Source: CAD feature listing. Evaluate the final solid. Frame: model axes, mm. A direction names the side the tool comes from. Give positions to 0.01 mm unless a question says otherwise; leave off trailing zeros. Write each loop counter-clockwise with the first axis right and the second up, starting at its lowest first coordinate (ties: lowest second). Pieces come first, ordered by that corner, then holes. Notation, with made-up numbers: (46.25, 7) -> (70.25, 7) arc R20 ccw to (70.25, 12) -> close; hole circle Ø3 at (89.5, 79.25). An arc over 180 degrees is marked (long way). Answer as a JSON object with one key per item and string values. Group by question number.
Item 1: Pull-direction query (X, two-part tool) for faces 1 (the face through (0, 15, 33)), 2 (the face through (-25, 0, 50)), 3 (the face through (-14.985, -0.66, 14.79)); classes: pulls with the +X half, pulls with the -X half, needs draft (parallel to the pull), parting line crosses it, or undercut.
Item 2: Section query D-D on z = 26. Return the cut outline in (x, y), plus the area to 3 significant figures.
Item 3: Access query for faces 4 (the face through (0, 0, 35)), 5 (the face through (-30, 0, 47)), 6 (the face through (21, 0, 30)). Directions: +Z, -Z, +X, -X, +Y, -Y. A direction counts if a zero-diameter tool reaches every point of the face in a straight line with its end or side. Return the directions, or none.
Item 4: First-contact query: pin 1 Ø5 at (x, y) = (-18, -10.5) entering from -Z; pin 2 Ø2 at (x, y) = (-23.5, 10.5) entering from +Z. Flat tips, straight axial feed; report the tip coordinate or a pass-through.
Item 5: Section query C-C on x = -14. Return the cut outline in (y, z), plus the area to 3 significant figures.
Item 6: Section query A-A on z = 40. Return the cut outline in (x, y).
Item 7: Section query B-B on y = 0. Return the cut outline in (x, z).
Item 8: Ray query, probe 1 along X at (y, z) = (-1.5, 52.5); probe 2 along Z at (x, y) = (1, -3); probe 3 along Z at (x, y) = (19, 5.75). Return the intervals inside material, ascending. Write a range as from..to.
Autodesk Inventor part; units mm, degrees
ref_plane "YZ Plane" through (0, 0, 0) normal (1, 0, 0) x (0, 1, 0)
ref_plane "XZ Plane" through (0, 0, 0) normal (0, 1, 0) x (-1, 0, 0)
ref_plane "XY Plane" through (0, 0, 0) normal (0, 0, 1) x (1, 0, 0)
sketch "스케치1" plane through (0, 0, 0) normal (0, 0, 1) x (1, 0, 0)
  circle A0 centre (0, 0) radius 15
  dimension "d0" = 30
extrude "돌출1" add sketch "스케치1" along normal blind 30
sketch "스케치2" plane through (0, 0, 30) normal (0, 0, 1) x (1, 0, 0)
  line L0 (30, 15) -> (-30, 15)
  line L1 (-30, 15) -> (-30, -15)
  line L2 (-30, -15) -> (30, -15)
  line L3 (30, -15) -> (30, 15)
  line L4 (30, 15) -> (-30, -15) construction
  line L5 (-30, 15) -> (30, -15) construction
  point P0 (0, 0)
  dimension "d3" = 60
  dimension "d4" = 30
extrude "돌출2" add sketch "스케치2" along normal blind 5
sketch "스케치3" plane through (30, -15, 30) normal (1, 0, 0) x (0, 0, -1)
  line L0 (0, 0) -> (0, 30)
  line L1 (0, 30) -> (-5, 30)
  line L2 (-5, 0) -> (-5, 30)
  line L3 (0, 0) -> (-5, 0)
  line L4 (-5, 0) -> (-20, 0)
  line L5 (-20, 30) -> (-5, 30)
  line L6 (-5, 30) -> (-5, 0)
  line L7 (0, 0) -> (-5, 0)
  line L8 (0, 30) -> (-5, 30)
  arc A0 (-20, 30) -> (-20, 0) centre (-20, 15) ccw
  point P0 (30, 15)
  dimension "d10" = 15
  dimension "d11" = 15
  dimension "d12" = 15
extrude "돌출3" add sketch "스케치3" against normal blind 5 contours L4 A0 L5 L2
mirror "미러1" about plane through (0, 0, 0) normal (1, 0, 0) of "돌출3"
ref_plane "작업 평면1" through (0, 0, 0) normal (1, 0, 0) x (0, 1, 0)
properties part number "L1_0.1" material "ABS 플라스틱"
Worked answers:
{
 "1": {"face 1": "needs draft", "face 2": "undercut", "face 3": "parting line crosses it"},
 "2": {"outline": "circle Ø30 at (0, 0)", "area": "707 mm^2"},
 "3": {"face 4": "+Z, +Y, -Y", "face 5": "+Z, -Z, -X, +Y, -Y", "face 6": "-Z, +X"},
 "4": {"pin 1": "z = 30", "pin 2": "z = 35"},
 "5": {"outline": "(-15, 30) -> (-5.39, 30) -> (-5.39, 0) -> (5.39, 0) -> (5.39, 30) -> (15, 30) -> (15, 35) -> (-15, 35) -> close", "area": "473 mm^2"},
 "6": {"outline": "(-30, -15) -> (-25, -15) -> (-25, 15) -> (-30, 15) -> close; (25, -15) -> (30, -15) -> (30, 15) -> (25, 15) -> close"},
 "7": {"outline": "(-30, 30) -> (-15, 30) -> (-15, 0) -> (15, 0) -> (15, 30) -> (30, 30) -> (30, 65) -> (25, 65) -> (25, 35) -> (-25, 35) -> (-25, 65) -> (-30, 65) -> close"},
 "8": {"probe 1": "-30..-25, 25..30", "probe 2": "0..35", "probe 3": "30..35"}
}
